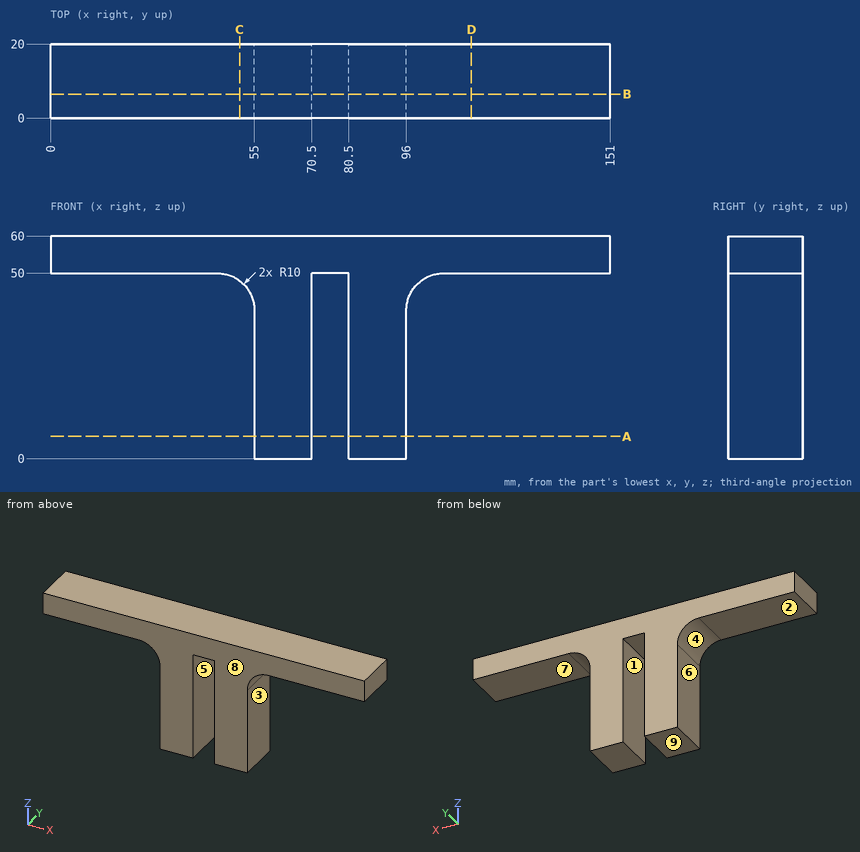
Input: dimensioned drawing with shaded views. Units: mm. Origin: part minimum x, y, z. A direction names the side the tool comes from. Round coordinates to 2 decimals unless told otherwise and drop trailing zeros. Order: outer loops, then holes, each group sorted by start corner. A loop starts at its lowest first (then second) coordinate and runs counter-clockwise, first axis right, second up. Notation, with made-up numbers: (60, -37) - (107, -37) arc R15 cw to (107, -10) - close; hole circle Ø6 at (68, 27). An arc over 180 degrees is marked (long way). Use CSV: the item, a comma, the result in double quotes. Start each with the question number.
Q1. First-contact query: pin 1 (10 mm diameter, centred on y = 10.5, z = 19, fed in from -X); pin 2 (10 mm diameter, centred on y = 11, z = 17, fed in from +X); pin 3 (5 mm diameter, centred on y = 13.5, z = 46.5, fed in from -X). Flat tips, straight axial feed; report the tip coordinate or a pass-through.
Q2. Mould query, pull axis X, two halves, no side actions, for the marked faces 1, 2, 3 and 4. Classes: +X half, -X half, draft (parallel to the pull), parting line (faces both ways), or undercut.
Q3. Section query C-C (x = 51). Return loops of the section in (y, z), and give its area (3 significant figures).
Q4. Section query D-D (x = 113.5). Return loops of the section in (y, z).
Q5. Section query B-B (y = 6.5). Return loops of the section in (x, z).
Q6. Access query for the marked faces 5, 6, 7, 8 and 9. Directions: +Z, -Z, +X, -X, +Y, -Y. A direction counts if a zero-diameter tool reaches every point of the face in a straight line with its end or side. Return the directions, or none.
Q7. Section query A-A (z = 6). Return loops of the section in (x, y).
Q8. Material intervals for line 1 along X through (y, z) = (10.5, 23); line 2 along Z through (x, y) = (78, 5); line 3 along Z through (x, y) = (53, 2.75), sorted ascending. Write a range as from..to.
Result set:
1,pin 1,"stops at x = 55"
1,pin 2,"stops at x = 96"
1,pin 3,"stops at x = 49.36"
2,face 1,"undercut"
2,face 2,"draft"
2,face 3,"+X half"
2,face 4,"-X half"
3,outline,"(0, 48) - (20, 48) - (20, 60) - (0, 60) - close"
3,area,"240 mm2"
4,outline,"(0, 50) - (20, 50) - (20, 60) - (0, 60) - close"
5,outline,"(0, 50) - (45, 50) arc R10 cw to (55, 40) - (55, 0) - (70.5, 0) - (70.5, 50) - (80.5, 50) - (80.5, 0) - (96, 0) - (96, 40) arc R10 cw to (106, 50) - (151, 50) - (151, 60) - (0, 60) - close"
6,face 5,"-Z, +Y, -Y"
6,face 6,"-Z, -X, +Y, -Y"
6,face 7,"-Z, +X, +Y, -Y"
6,face 8,"+Z, -Z, +X, -X, -Y"
6,face 9,"-Z, +X, -X, +Y, -Y"
7,outline,"(55, 0) - (70.5, 0) - (70.5, 20) - (55, 20) - close; (80.5, 0) - (96, 0) - (96, 20) - (80.5, 20) - close"
8,line 1,"x = 55..70.5, 80.5..96"
8,line 2,"z = 50..60"
8,line 3,"z = 46..60"
